Could you check a few things on this model? Use its own coordinates, in mm. A direction names the side the tool comes from. Give positions to 0.01 mm unless a question says otherwise; leave off trailing zeros. Loops run counter-clockwise (first coordinate to the right, second up) from the corner with the lowest first, then second, coordinate; pieces in that order, holes last. Notation, with made-up numbers: M -19.5,17 L 28.5,17 A14 ccw 28.5,44 Z; hole C 50.25,40.25 d7. An arc over 180 degrees is marked long. Use CSV: the item, a comma, the result in double quotes.
```python
from build123d import *

# Parameters (mm, degrees)
SKIZZE1_W                       = 275
SKIZZE1_H                       = 80
AUFSATZ_LINEAR_AUSTRAGEN1_DEPTH = 5
SKIZZE2_W                       = 100
SKIZZE2_H                       = 5
AUFSATZ_LINEAR_AUSTRAGEN2_DEPTH = 5
SKIZZE3_W                       = 5
SKIZZE3_H                       = 40
AUFSATZ_LINEAR_AUSTRAGEN3_DEPTH = 5


with BuildPart() as part:
    # Skizze1 → Aufsatz-Linear austragen1 (new body)
    with BuildSketch(Plane.XY):
        with Locations((137.5, 40)):
            Rectangle(SKIZZE1_W, SKIZZE1_H)
    extrude(amount=AUFSATZ_LINEAR_AUSTRAGEN1_DEPTH)

    # Skizze2 → Aufsatz-Linear austragen2 (add, through all)
    with BuildSketch(Plane.XY.offset(5)):
        with Locations((137.5, -2.5)):
            Rectangle(SKIZZE2_W, SKIZZE2_H)
    extrude(amount=-AUFSATZ_LINEAR_AUSTRAGEN2_DEPTH)

    # Skizze3 → Aufsatz-Linear austragen3 (add, through all)
    with BuildSketch(Plane.XY.offset(5)):
        with Locations((-2.5, 40)):
            Rectangle(SKIZZE3_W, SKIZZE3_H)
        with Locations((277.5, 40)):
            Rectangle(SKIZZE3_W, SKIZZE3_H)
    extrude(amount=-AUFSATZ_LINEAR_AUSTRAGEN3_DEPTH)


solid = part.part
```
1. I'm going to push flat-ended pins straight in: pin 1 Ø1.5 at (y, z) = (5.5, 2) entering from +X; pin 2 Ø1.5 at (x, z) = (277.5, 3) entering from +Y; pin 3 Ø1.5 at (y, z) = (-2, 3) entering from -X. Where does each tip first touch, or does it pass through?
Outcome:
pin 1,"x = 275"
pin 2,"y = 60"
pin 3,"x = 87.5"
2. I want a section at C-C, the plane y = 71. List the corners of the cut face in (x, z) for me, then the cut area to 4 significant figures.
Outcome:
outline,"M 0,0 L 275,0 L 275,5 L 0,5 Z"
area,"1,375 mm2"
3. I want a section at B-B, the plane x = 83. List the corners of the cut face in (y, z) for me.
Outcome:
outline,"M 0,0 L 80,0 L 80,5 L 0,5 Z"
4. Please list where these lines run through material, in increasing order: line 1 (Y direction, x = 188, z = 4.6); line 2 (X direction, y = 1.5, z = 0.35).
Outcome:
line 1,"0 to 80"
line 2,"0 to 275"
5. I want a section at A-A, the plane z = 2.8. List the corners of the cut face in (x, y) for me, then the cut area to 3 significant figures.
Outcome:
outline,"M -5,20 L 0,20 L 0,0 L 87.5,0 L 87.5,-5 L 187.5,-5 L 187.5,0 L 275,0 L 275,20 L 280,20 L 280,60 L 275,60 L 275,80 L 0,80 L 0,60 L -5,60 Z"
area,"22,900 mm2"
6. Which directions (+Z, -Z, +X, -X, +Y, -Y) give clear straight access to the entire face, cutting with the end or side of a thin tool? Please do faces 1 (the face through (187.5, -3, 3)), 2 (the face through (280, 40, 3)), 3 (the face through (275, 70, 2)), 4 (the face through (87.5, -3, 3)), 5 (the face through (0, 70, 2)).
Outcome:
face 1,"+Z, -Z, +X, -Y"
face 2,"+Z, -Z, +X, +Y, -Y"
face 3,"+Z, -Z, +X, +Y"
face 4,"+Z, -Z, -X, -Y"
face 5,"+Z, -Z, -X, +Y"
